Could you check a few things on this model? Use its own coordinates, in mm. Face numbers are marked on the shaded views. A direction names the side the tool comes from. Round coordinates to 2 decimals unless told otherwise and drop trailing zeros. Loops run counter-clockwise (first coordinate to the right, second up) from the corner with the lowest first, then second, coordinate; pieces in that order, holes last. Notation, with made-up numbers: (-36, 55.5) -> (17, 55.5) arc R25 ccw to (17, 80.5) -> close; hole circle Ø7 at (13.5, -4). An arc over 180 degrees is marked (long way). Put each result on its own line as item: value. Start each with the question number.
1. I'm going to push flat-ended pins straight in: P1, Ø1.5, axis at y = 49.5, z = 3, coming from the +X side; P2, Ø5, axis at x = 3.5, y = 59, coming from the -Z side; P3, Ø6, axis at y = 23.5, z = -2.5, coming from the -X side; P4, Ø10, axis at x = 16.5, z = 13.5, coming from the -Y side. Where does each tip first touch, or does it pass through?
2. I need wall thicknesses on line 1 (Y direction, x = -17, z = 10); line 2 (Z direction, x = 8.5, y = 31); line 3 (X direction, y = 25, z = 9). Which ranges of each line are inside material? Lowest first, please. Write a range as [from, to].
3. Which directions (+Z, -Z, +X, -X, +Y, -Y) give clear straight access to the entire face, cutting with the end or side of a thin tool? Please do the marked faces 1, 2, 3, 4 and 5.
4. Imagine slicing it at C-C, the plane y = 43.5. Please give me the cut outline in (x, z).
5. Imagine slicing it at D-D, the plane y = 29. Please give me the cut outline in (x, z), and give its area (3 significant figures).
6. Imagine slicing it at B-B, the plane x = 0. Please give me the cut outline in (y, z).
7. Imagine slicing it at A-A, the plane z = 16. Please give me the cut outline in (x, y).
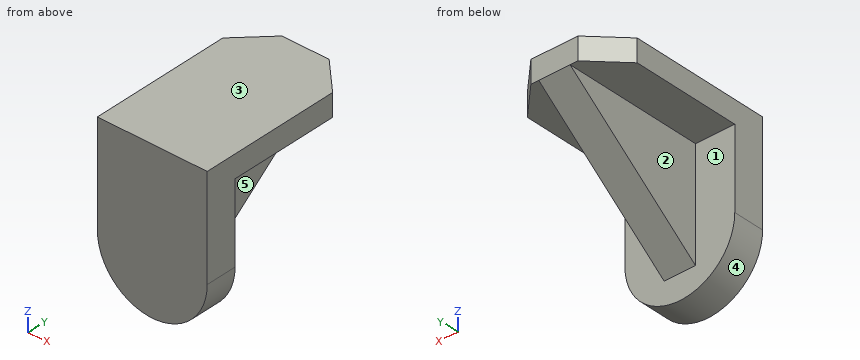
```python
from build123d import *

# Parameters (mm, degrees)
SKETCH1_W           = 42
SKETCH1_H           = 39
BOSS_EXTRUDE1_DEPTH = 12
SKETCH2_W           = 42
SKETCH2_H           = 8.570511372
BOSS_EXTRUDE2_DEPTH = 54
CHAMFER1_SIZE       = 12
BOSS_EXTRUDE3_DEPTH = 6


with BuildPart() as part:
    # Sketch1 → Boss-Extrude1 (new body)
    with BuildSketch(Plane(origin=(0, 0, 0), x_dir=(1, 0, 0), z_dir=(0, 1, 0))):
        Rectangle(SKETCH1_W, SKETCH1_H)
        with BuildLine():
            ThreePointArc((-21, 19.5), (0, 40.5), (21, 19.5))
            Line((21, 19.5), (-21, 19.5))
        make_face()
    extrude(amount=BOSS_EXTRUDE1_DEPTH)

    # Sketch2 → Boss-Extrude2 (add)
    with BuildSketch(Plane(origin=(0, 12, 0), x_dir=(1, 0, 0), z_dir=(0, 1, 0))):
        with Locations((0, -15.214744314)):
            Rectangle(SKETCH2_W, SKETCH2_H)
    extrude(amount=BOSS_EXTRUDE2_DEPTH)

    # Chamfer1
    chamfer1_edges = [part.edges().sort_by_distance(p)[0] for p in [
        (-21, 66, 15.214744314),
        (21, 66, 15.214744314),
    ]]
    chamfer(chamfer1_edges, length=CHAMFER1_SIZE)

    # Sketch5 → Boss-Extrude3 (add, symmetric)
    with BuildSketch(Plane(origin=(0, 0, 0), x_dir=(0, 0, -1), z_dir=(1, 0, 0))):
        Polygon((-10.929488628, 66), (-10.929488628, 12), (31.070511372, 12), align=None)
    extrude(amount=BOSS_EXTRUDE3_DEPTH, both=True)


solid = part.part
```
Entries:
1. P1: x = 6
1. P2: z = 3.54
1. P3: x = -6
1. P4: y = 0
2. line 1: [0, 12]
2. line 2: [10.93, 19.5]
2. line 3: [-6, 6]
3. face 1: -Z, +Y
3. face 2: -Z, -X, +Y
3. face 3: +Z, +X, -X, +Y, -Y
3. face 4: -Z, +Y, -Y
3. face 5: -Z, +X, +Y
4. outline: (-21, 10.93) -> (-6, 10.93) -> (-6, -6.57) -> (6, -6.57) -> (6, 10.93) -> (21, 10.93) -> (21, 19.5) -> (-21, 19.5) -> close
5. outline: (-21, 10.93) -> (-6, 10.93) -> (-6, -17.85) -> (6, -17.85) -> (6, 10.93) -> (21, 10.93) -> (21, 19.5) -> (-21, 19.5) -> close
5. area: 705 mm^2
6. outline: (0, -40.5) -> (12, -40.5) -> (12, -31.07) -> (66, 10.93) -> (66, 19.5) -> (0, 19.5) -> close
7. outline: (-21, 0) -> (21, 0) -> (21, 54) -> (9, 66) -> (-9, 66) -> (-21, 54) -> close
